The listing builds one solid part. Answer for the finished solid, in the listing's coordinates (mm). Face numbers are marked on the shaded views. A direction names the side the tool comes from. Coordinates: 2 decimals unless noted, no trailing zeros. Order: outer loops, then holes, each group sorted by start corner. A loop starts at its lowest first (then second) coordinate and runs counter-clockwise, first axis right, second up. Notation, with made-up numbers: (79, -17.75) - (133, -17.75) arc R20 ccw to (133, -0.75) - close; hole circle Ø1 at (4, -9). An arc over 180 degrees is marked (long way). One line per item, written item: value. Start each with the question number.
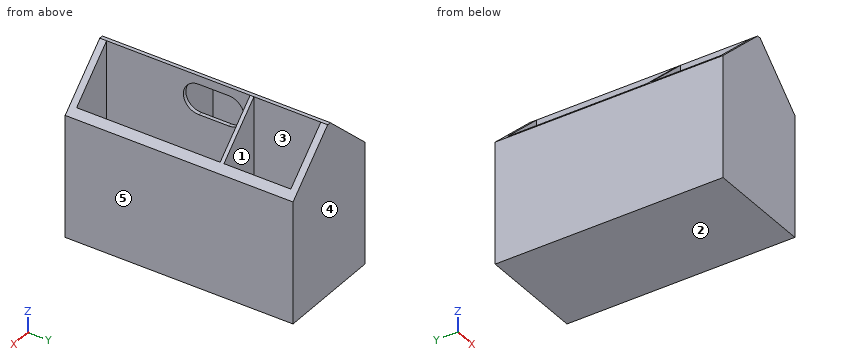
```python
from build123d import *

# Parameters (mm, degrees)
F0_W     = 88.9
F0_H     = 190.5
F0_W_2   = 82.55
F0_H_2   = 184.15
F1_DEPTH = 3.175
F2_W     = 88.9
F2_H     = 190.5
F2_W_2   = 3.175
F2_H_2   = 3.175
F2_W_3   = 37.1475
F2_H_3   = 58.1914
F2_H_4   = 55.9145467066
F2_H_5   = 58.6140532934
F3_DEPTH = 139.7
F6_DEPTH = 190.5
F8_DEPTH = 25.4


# Not quite as in the source:
# - a feature names something its author has since deleted; it is built from what else it names


with BuildPart() as f1:
    # F0 (on Top) → F1 (new body)
    with BuildSketch(Plane.XY):
        Rectangle(F0_W, F0_H)
        Rectangle(F0_W_2, F0_H_2, mode=Mode.SUBTRACT)
        Rectangle(F0_W_2, F0_H_2)
    extrude(amount=F1_DEPTH)

    # F2 (on face) → F3 (join)
    with BuildSketch(Plane.XY.offset(3.175)):
        Rectangle(F2_W, F2_H)
        Polygon((-1.5875, -89.535), (-38.735, -89.535), (-38.735, -30.9209467066), (-38.735, -27.7459467066), (-38.735, 89.535), (-1.5875, 89.535), (1.5875, 89.535), (38.735, 89.535), (38.735, 33.6204532934), (38.735, 30.4454532934), (38.735, -89.535), (1.5875, -89.535), align=None, mode=Mode.SUBTRACT)
        with Locations((0, 32.0329532934)):
            Rectangle(F2_W_2, F2_H_2)
        with Locations((20.16125, 32.0329532934)):
            Rectangle(F2_W_3, F2_H_2)
        with Locations((-20.16125, -29.3334467066)):
            Rectangle(F2_W_3, F2_H_2)
        with Locations((0, -29.3334467066)):
            Rectangle(F2_W_2, F2_H_2)
        with Locations((0, 1.3497532934)):
            Rectangle(F2_W_2, F2_H_3)
        with Locations((0, 61.5777266467)):
            Rectangle(F2_W_2, F2_H_4)
        with Locations((0, -60.2279733533)):
            Rectangle(F2_W_2, F2_H_5)
    extrude(amount=F3_DEPTH)

    # F5 (on face) → F6 (cut)
    with BuildSketch(Plane.XZ.offset(95.25)):
        Polygon((-44.45, 102.3109257221), (-1.5860880958, 142.875), (-44.45, 142.875), align=None)
        Polygon((44.45, 142.875), (1.5860880958, 142.875), (44.45, 102.3109257221), align=None)
    extrude(amount=-F6_DEPTH, mode=Mode.SUBTRACT)

    # F7 (on face) → F8 (cut)
    with BuildSketch(Plane.YZ.offset(1.5875)):
        with BuildLine():
            Line((12.7, 135.732749784), (0, 135.732749784))
            Line((0, 135.732749784), (-12.7, 135.732749784))
            ThreePointArc((-12.7, 135.732749784), (-25.4008333473, 122.8855821986), (-12.4090174213, 110.332749784))
            Line((-12.4090174213, 110.332749784), (0, 110.332749784))
            Line((0, 110.332749784), (12.4090174213, 110.332749784))
            ThreePointArc((12.4090174213, 110.332749784), (25.4008333473, 122.8855821986), (12.7, 135.732749784))
        make_face()
    extrude(amount=-F8_DEPTH, mode=Mode.SUBTRACT)


solid = f1.part
```
(1) For a pull along Y with two mould halves and no side action, classify the marked faces 3, 4 and 5 as pulls with the +Y half, pulls with the -Y half, needs draft (parallel to the pull), parting line crosses it, or undercut.
(2) For the marked faces 1 and 2, determine the directions among +Z, -Z, +X, -X, +Y, -Y from which every point of the face is accessible in a straight line to the end or side of a thin tool.
(3) A flat-ended cylindrical pin translates along its axis: pin 1 Ø11 at (x, y) = (-21.5, 43) entering from +Z (3 decimals). Find the tip coordinate at first contact, or state that the pin passes through.
(4) The part is cut by section A-A on z = 53. Count the separate pieces of the cut face and the enclosed holes in it, plus the area to 3 significant figures.
(5) Consider probe 1 along Y at (x, z) = (-24.5, 110.5) (3 decimals); probe 2 along Y at (x, z) = (4.5, 41) (3 decimals); probe 3 along Z at (x, y) = (-3, -79) (3 decimals). Determine where each line is inside the solid, lowest interval first.
(6) The part is cut by section D-D on x = 31.5. Determine the outline of the cut face in (y, z) (3 decimals).
Completed:
1. face 3: undercut
1. face 4: pulls with the +Y half
1. face 5: needs draft
2. face 1: +Z
2. face 2: -Z, +X, -X, +Y, -Y
3. pin 1: stops at z = 3.175
4. separate pieces: 1
4. enclosed holes: 4
4. area: 3,870 mm2
5. probe 1: y = -95.25 to -89.535, -30.921 to -27.746, 89.535 to 95.25
5. probe 2: y = -95.25 to -89.535, 30.445 to 33.62, 89.535 to 95.25
5. probe 3: z = 0 to 3.175
6. outline: (-95.25, 0) - (95.25, 0) - (95.25, 114.566) - (89.535, 114.566) - (89.535, 3.175) - (33.62, 3.175) - (33.62, 114.566) - (30.445, 114.566) - (30.445, 3.175) - (-89.535, 3.175) - (-89.535, 114.566) - (-95.25, 114.566) - close
